from build123d import *

# Parameters (mm, degrees)
SKETCH1_R           = 9
SKETCH1_R_2         = 1.6
BOSS_EXTRUDE1_DEPTH = 3
BOSS_EXTRUDE2_DEPTH = 10
SKETCH3_R           = 9
BOSS_EXTRUDE3_DEPTH = 25
BOSS_EXTRUDE3_TAPER = 10
SKETCH4_R           = 4.591825482
BOSS_EXTRUDE4_DEPTH = 25


with BuildPart() as part:
    # Sketch1 → Boss-Extrude1 (new body)
    with BuildSketch(Plane(origin=(0, 0, 0), x_dir=(1, 0, 0), z_dir=(0, 1, 0))):
        Circle(SKETCH1_R)
        Circle(SKETCH1_R_2, mode=Mode.SUBTRACT)
    boss_extrude1 = extrude(amount=BOSS_EXTRUDE1_DEPTH)

    # Sketch2 → Boss-Extrude2 (add)
    with BuildSketch(Plane.XZ):
        with BuildLine():
            Line((-7.483314774, 5), (0, 5))
            ThreePointArc((0, 5), (3.535533906, 3.535533906), (5, 0))
            ThreePointArc((5, 0), (3.535533906, -3.535533906), (0, -5))
            Line((0, -5), (-7.483314774, -5))
            ThreePointArc((-7.483314774, -5), (2.61248608, -8.61248608), (9, 0))
            ThreePointArc((9, 0), (2.61248608, 8.61248608), (-7.483314774, 5))
        make_face()
    boss_extrude2 = extrude(amount=BOSS_EXTRUDE2_DEPTH)

    # Sketch3 → Boss-Extrude3 (add)
    with BuildSketch(Plane.XZ.offset(10)):
        Circle(SKETCH3_R)
    boss_extrude3 = extrude(amount=BOSS_EXTRUDE3_DEPTH, taper=BOSS_EXTRUDE3_TAPER)

    # Sketch4 → Boss-Extrude4 (add)
    with BuildSketch(Plane.XZ.offset(35)):
        Circle(SKETCH4_R)
    boss_extrude4 = extrude(amount=BOSS_EXTRUDE4_DEPTH)

    # Mirror2: Boss-Extrude1, Boss-Extrude2, Boss-Extrude3, Boss-Extrude4 across plane
    add(boss_extrude1.mirror(Plane(origin=(0, -60, 0), x_dir=(0, 0, 1), z_dir=(0, -1, 0))))
    add(boss_extrude2.mirror(Plane(origin=(0, -60, 0), x_dir=(0, 0, 1), z_dir=(0, -1, 0))))
    add(boss_extrude3.mirror(Plane(origin=(0, -60, 0), x_dir=(0, 0, 1), z_dir=(0, -1, 0))))
    add(boss_extrude4.mirror(Plane(origin=(0, -60, 0), x_dir=(0, 0, 1), z_dir=(0, -1, 0))))


solid = part.part
CAD build for the part. Positions are in the model's coordinates, mm. A direction names the side the tool comes from. Give positions to 0.01 mm unless a question says otherwise; leave off trailing zeros. Loops run counter-clockwise (first coordinate to the right, second up) from the corner with the lowest first, then second, coordinate; pieces in that order, holes last. Notation, with made-up numbers: M -16.5,-29 L -4.5,-29 A22 ccw -4.5,-2 Z; hole C 86.5,-13 d1. An arc over 180 degrees is marked long. Write each question's results on one line, items separated by ' | '.
Q1. Band-saw the part on B-B on x = -3.5. Give the number of separate pieces and of enclosed holes in the cut face, and give its area (3 significant figures).
Geometry check:
separate pieces: 1 | enclosed holes: 2 | area: 1,110 mm²
Q2. Band-saw the part on A-A on y = -62. Write the cut outline in (x, z), and give its area (3 significant figures).
Geometry check:
outline: C 0,0 d9.18 | area: 66.2 mm²
Q3. Flat gauge pins, fed straight in: P1, Ø5, axis at x = 3, y = -39, coming from the -Z side; P2, Ø6, axis at x = -4, y = -113, coming from the -Z side; P3, Ø2.5, axis at x = 0, z = 0, coming from the +Y side; P4, Ø8, axis at x = -2, y = -5, coming from the +Z side. Where does each tip first touch, or does it go through?
Geometry check:
P1: stops at z = -4.56 | P2: stops at z = -8.94 | P3: stops at y = -10 | P4: stops at z = 9
Q4. Mould opens along Z. For faces 4 (the face through (-2, -110, 0)), 5 (the face through (0, 3, 2)), 6 (the face through (6.453, -97.325, 2.032)) say: pulls with the +Z half, pulls with the -Z half, needs draft (parallel to the pull), parting line crosses it, or undercut.
Geometry check:
face 4: undercut | face 5: needs draft | face 6: parting line crosses it
Q5. Probe probe 1 along Y at (x, z) = (-3.5, -2.5); probe 2 along Z at (x, y) = (0, 1.45). List the from-to ranges inside material, lowest first.
Geometry check:
probe 1: y = -123 to -120, -110 to -10, 0 to 3 | probe 2: z = -9 to -1.6, 1.6 to 9
Q6. Band-saw the part on C-C on y = -88. Write the cut outline in (x, z), and give its area (3 significant figures).
Geometry check:
outline: C 0,0 d10.24 | area: 82.4 mm²
Q7. Which spindle directions (+Z, -Z, +X, -X, +Y, -Y) get a long thin tool onto all of the face, cutting with end or side? Do faces 1 (the face through (-1.27, 1.48, 0.97)), 2 (the face through (6.453, -22.675, 2.032)), 3 (the face through (-2, -120, 0)). Say none if no direction does.
Geometry check:
face 1: +Y | face 2: none | face 3: -X
